from build123d import *

# Parameters (mm, degrees)
F0_W     = 44.45
F0_H     = 25.4
F1_DEPTH = 63.5


with BuildPart() as f1:
    # F0 (on Front) → F1 (new body, symmetric)
    with BuildSketch(Plane.XZ):
        Polygon((0, 82.55), (-63.5, 82.55), (-63.5, 0), (63.5, 0), (63.5, 82.55), (44.45, 82.55), (44.45, 57.15), (0, 57.15), align=None)
        with Locations((22.225, 69.85)):
            Rectangle(F0_W, F0_H)
    extrude(amount=F1_DEPTH, both=True)

    # F0 (on Front) → F2 (revolve, cut)
    with BuildSketch(Plane.XZ):
        with Locations((22.225, 69.85)):
            Rectangle(F0_W, F0_H)
    revolve(axis=Axis((0, 0, 41.275), (0, 0, 1)), mode=Mode.SUBTRACT)


solid = f1.part
Design review of the part built by this model. Coordinates are the model's own, in mm. A direction names the side the tool comes from. Coordinates: 2 decimals unless noted, no trailing zeros. Write each loop counter-clockwise with the first axis right and the second up, starting at its lowest first coordinate (ties: lowest second). Pieces come first, ordered by that corner, then holes. Notation, with made-up numbers: (-29, -26.5) -> (11, -26.5) arc R12 cw to (11, -12.5) -> close; hole circle Ø5 at (-23, -14.5). An arc over 180 degrees is marked (long way). Write each question's results on one line, items separated by ' | '. Start each with the question number.
(1) Clearance check with a flat-ended pin moving along its axis: P1, Ø12, axis at x = -13, y = 19, coming from the +Z side. State where the tip first meets the part, or that it passes through.
(2) Tool access review of faces 5 (the face through (43, -15, 82.55)), 6 (the face through (1, 1, 57.15)): name each direction out of +Z, -Z, +X, -X, +Y, -Y from which nothing blocks a thin tool from reaching the whole face with its end or side.
(3) Take a section at A-A on x = 0. Write out the cut boundary in (y, z), and give its area (3 significant figures).
(4) For line 1 along Y through (x, z) = (0, 64.25); line 2 along Z through (x, y) = (-1.5, -8.5); line 3 along X through (y, z) = (5, 77), list the stretches that pass through material, from the lowest coordinate up. Write a range as from..to.
(5) The part is to be moulded in two halves that separate along X. For faces 1 (the face through (42.397, 13.352, 70.028)), 2 (the face through (-1, 63.5, 42)), 3 (the face through (-63.5, -1, 42)), 4 (the face through (63.5, -1, 41)), say which applies: pulls with the +X half, pulls with the -X half, needs draft (parallel to the pull), parting line crosses it, or undercut.
(6) Take a section at B-B on z = 70. Write out the cut boundary in (x, y).
Results found:
1) P1: stops at z = 57.15
2) face 5: +Z, +X, -X, +Y, -Y | face 6: +Z
3) outline: (-63.5, 0) -> (63.5, 0) -> (63.5, 82.55) -> (44.45, 82.55) -> (44.45, 57.15) -> (-44.45, 57.15) -> (-44.45, 82.55) -> (-63.5, 82.55) -> close | area: 8,230 mm2
4) line 1: y = -63.5..-44.45, 44.45..63.5 | line 2: z = 0..57.15 | line 3: x = -63.5..-44.17, 44.17..63.5
5) face 1: undercut | face 2: needs draft | face 3: pulls with the -X half | face 4: pulls with the +X half
6) outline: (-63.5, -63.5) -> (63.5, -63.5) -> (63.5, 63.5) -> (-63.5, 63.5) -> close; hole circle Ø88.9 at (0, 0)
